The listing builds one solid part. Answer for the finished solid, in the listing's coordinates (mm). A direction names the side the tool comes from. Coordinates: 2 decimals unless noted, no trailing zeros. Loops run counter-clockwise (first coordinate to the right, second up) from the corner with the lowest first, then second, coordinate; pieces in that order, holes last. Notation, with made-up numbers: (70.5, 30) - (98.5, 30) arc R22 ccw to (98.5, 38) - close; hole circle Ø7 at (-33, 10.25). An arc over 180 degrees is marked (long way). Return JSON: item names as keys, results as strings. Group by question number.
1. Each of these flat-tipped pins is pushed along its axis until it touches: P1, Ø2, axis at x = -13, y = 13.5, coming from the +Z side; P2, Ø0.8, axis at x = 16.5, z = 34.5, coming from the -Y side; P3, Ø5, axis at x = 12, y = 12.5, coming from the -Z side. Where does it stop, or does it pass through?
2. Section D-D (x = -4.5) is taken. Write down the section's boundary in (y, z), and give its area (3 significant figures).
3. Section B-B (x = 0) is taken. Write down the section's boundary in (y, z), and give its area (4 significant figures).
4. Which of the six approach directions +Z, -Z, +X, -X, +Y, -Y give full straight-line access (tool end or side, diameter ignored) to faces 4 (the face through (9.605, -9.803, 2.218)), 5 (the face through (-9.88, -11.23, 45)), 6 (the face through (10.316, 7.91, 2.24)), 7 (the face through (-15.03, 7.714, 24.404)), 8 (the face through (-15.028, 2.082, 41.977))?
5. Find the intervals of material crossed by line 1 along Z through (x, y) = (6, 11); line 2 along Y through (x, z) = (-10.5, 24.5); line 3 along X through (y, z) = (-8.5, 15), in increasing order.
6. Section C-C (z = 30.5) is taken. State how many separate pieces and enclosed holes the cut face has, and give its area (3 significant figures).
7. The mould has two halves that part along Y. Classify faces 1 (the face through (3.5, -16, 24)), 2 (the face through (13.805, 1, 24)), 3 (the face through (-9, -17, 24)): pulls with the +Y half, pulls with the -Y half, needs draft (parallel to the pull), parting line crosses it, or undercut.
```python
from build123d import *

# Parameters (mm, degrees)
SKETCH_1_R          = 12.5
SKETCH_1_R_2        = 2.1
EXTRUDE_1_DEPTH     = 49.5
SKETCH_2_R          = 3.25
CUT_EXTRUDE_2_DEPTH = 4.5
SKETCH_4_W          = 13
SKETCH_4_H          = 1.5
SKETCH_5_R          = 2.1
CUT_EXTRUDE_3_DEPTH = 4


with BuildPart() as part:
    # 草图1 → 拉伸1 (new body)
    with BuildSketch(Plane.XY):
        with BuildLine():
            Line((-17, 8.268803112), (-16.434277079, 8.730182715))
            Line((-16.434277079, 8.730182715), (-13.585223978, 6.669165578))
            Line((-13.585223978, 6.669165578), (-15.009750528, 4.699967111))
            Line((-15.009750528, 4.699967111), (-16.756503192, 5.963575421))
            Line((-16.756503192, 5.963575421), (-16.756503192, 6.669165578))
            Line((-16.756503192, 6.669165578), (-17, 6.669165578))
            Line((-17, 6.669165578), (-17, -6.669165578))
            Line((-17, -6.669165578), (-16.756503192, -6.669165578))
            Line((-16.756503192, -6.669165578), (-16.756503192, -5.963575421))
            Line((-16.756503192, -5.963575421), (-15.009750528, -4.699967111))
            Line((-15.009750528, -4.699967111), (-13.585223978, -6.669165578))
            Line((-13.585223978, -6.669165578), (-16.434277079, -8.730182715))
            Line((-16.434277079, -8.730182715), (-17, -8.268803112))
            Line((-17, -8.268803112), (-17, -14.739402973))
            ThreePointArc((-17, -14.739402973), (-15.909902577, -15.909902577), (-14.739402973, -17))
            Line((-14.739402973, -17), (-3.5, -17))
            Line((-3.5, -17), (-3.5, -14))
            Line((-3.5, -14), (4.42289808, -14))
            Line((4.42289808, -14), (4.42289808, -15))
            Line((4.42289808, -15), (3.5, -15))
            Line((3.5, -15), (3.5, -17))
            Line((3.5, -17), (14.739402973, -17))
            ThreePointArc((14.739402973, -17), (15.909902577, -15.909902577), (17, -14.739402973))
            Line((17, -14.739402973), (17, -3.5))
            Line((17, -3.5), (13.805038875, -3.5))
            Line((13.805038875, -3.5), (13.805038875, 5))
            Line((13.805038875, 5), (15.402519437, 5))
            Line((15.402519437, 5), (15.402519437, 3.7))
            Line((15.402519437, 3.7), (17, 3.7))
            Line((17, 3.7), (17, 14.739402973))
            ThreePointArc((17, 14.739402973), (15.909902577, 15.909902577), (14.739402973, 17))
            Line((14.739402973, 17), (3.5, 17))
            Line((3.5, 17), (3.5, 15))
            Line((3.5, 15), (4.42289808, 15))
            Line((4.42289808, 15), (4.42289808, 14))
            Line((4.42289808, 14), (-3.5, 14))
            Line((-3.5, 14), (-3.5, 17))
            Line((-3.5, 17), (-14.739402973, 17))
            ThreePointArc((-14.739402973, 17), (-15.909902577, 15.909902577), (-17, 14.739402973))
            Line((-17, 14.739402973), (-17, 8.268803112))
        make_face()
        Circle(SKETCH_1_R, mode=Mode.SUBTRACT)
        with Locations((12, 12)):
            Circle(SKETCH_1_R_2, mode=Mode.SUBTRACT)
        with Locations((-12, 12)):
            Circle(SKETCH_1_R_2, mode=Mode.SUBTRACT)
        with Locations((-12, -12)):
            Circle(SKETCH_1_R_2, mode=Mode.SUBTRACT)
        with Locations((12, -12)):
            Circle(SKETCH_1_R_2, mode=Mode.SUBTRACT)
    extrude(amount=EXTRUDE_1_DEPTH)

    # 草图2 → 拉伸2 (cut)
    with BuildSketch(Plane.XY.offset(49.5)):
        with Locations((-12, 12)):
            Circle(SKETCH_2_R)
        with Locations((12, 12)):
            Circle(SKETCH_2_R)
        with Locations((12, -12)):
            Circle(SKETCH_2_R)
        with Locations((-12, -12)):
            Circle(SKETCH_2_R)
    cut_extrude_2 = extrude(amount=-CUT_EXTRUDE_2_DEPTH, mode=Mode.SUBTRACT)

    # 草图4 → 切除-旋转1 (revolve, cut)
    with BuildSketch(Plane(origin=(0, 0, 0), x_dir=(1, 0, 0), z_dir=(0, 1, 0)), mode=Mode.PRIVATE) as cut_revolve_1_sk:
        with Locations((6.5, -2.25)):
            Rectangle(SKETCH_4_W, SKETCH_4_H)
        with Locations((6.5, -47.25)):
            Rectangle(SKETCH_4_W, SKETCH_4_H)
    revolve(cut_revolve_1_sk.sketch.rotate(Axis((0, 0, 0), (0, 0, 1)), 180), axis=Axis((0, 0, 0), (0, 0, 1)), mode=Mode.SUBTRACT)

    # 镜向1: 拉伸2 across plane
    add(cut_extrude_2.mirror(Plane.XY.offset(24.75)), mode=Mode.SUBTRACT)

    # 草图5 → 拉伸3 (cut)
    with BuildSketch(Plane.ZY.offset(17)):
        with Locations((7.25, 0)):
            Circle(SKETCH_5_R)
        with Locations((42.25, 0)):
            Circle(SKETCH_5_R)
    extrude(amount=-CUT_EXTRUDE_3_DEPTH, mode=Mode.SUBTRACT)


solid = part.part
```
The answers:
{
 "1": {"P1": "stops at z = 45", "P2": "stops at y = -15.72", "P3": "stops at z = 4.5"},
 "2": {"outline": "(-17, 0) - (-11.66, 0) - (-11.66, 1.5) - (-12.2, 1.5) - (-12.2, 3) - (-11.66, 3) - (-11.66, 46.5) - (-12.2, 46.5) - (-12.2, 48) - (-11.66, 48) - (-11.66, 49.5) - (-17, 49.5) - close; (11.66, 0) - (17, 0) - (17, 49.5) - (11.66, 49.5) - (11.66, 48) - (12.2, 48) - (12.2, 46.5) - (11.66, 46.5) - (11.66, 3) - (12.2, 3) - (12.2, 1.5) - (11.66, 1.5) - close", "area": "525 mm2"},
 "3": {"outline": "(-14, 0) - (-12.5, 0) - (-12.5, 1.5) - (-13, 1.5) - (-13, 3) - (-12.5, 3) - (-12.5, 46.5) - (-13, 46.5) - (-13, 48) - (-12.5, 48) - (-12.5, 49.5) - (-14, 49.5) - close; (12.5, 0) - (14, 0) - (14, 49.5) - (12.5, 49.5) - (12.5, 48) - (13, 48) - (13, 46.5) - (12.5, 46.5) - (12.5, 3) - (13, 3) - (13, 1.5) - (12.5, 1.5) - close", "area": "145.5 mm2"},
 "4": {"face 4": "-Z", "face 5": "+Z", "face 6": "none", "face 7": "+Z, -Z", "face 8": "-X"},
 "5": {"line 1": "z = 0 to 1.5, 3 to 46.5, 48 to 49.5", "line 2": "y = -17 to -13.47, -10.53 to -6.78, 6.78 to 10.53, 13.47 to 17", "line 3": "x = -17 to -16.72, -16.12 to -9.17, 9.17 to 17"},
 "6": {"separate pieces": "1", "enclosed holes": "5", "area": "516 mm2"},
 "7": {"face 1": "needs draft", "face 2": "undercut", "face 3": "pulls with the -Y half"}
}
